from build123d import *
from OCP.BRepFilletAPI import BRepFilletAPI_MakeChamfer

# Parameters (mm, degrees)
SKETCH_1_R          = 2.85
EXTRUDE_1_DEPTH     = 1.4
FILLET_1_R          = 1.4
SKETCH_3_R          = 1.5
EXTRUDE_3_DEPTH     = 8
CUT_EXTRUDE_1_DEPTH = 1
CHAMFER_2_SIZE      = 0.3
CHAMFER_3_SIZE      = 0.576368876
CHAMFER_3_SIZE2     = 0.998300177
FILLET_2_R          = 0.1


with BuildPart() as part:
    # 草图1 → 凸台-拉伸1 (new body)
    with BuildSketch(Plane.XY):
        Circle(SKETCH_1_R)
    extrude(amount=EXTRUDE_1_DEPTH)

    # 圆角1
    fillet_1_edges = [part.edges().sort_by_distance(p)[0] for p in [
        (-2.85, 0, 1.4),
    ]]
    fillet(fillet_1_edges, radius=FILLET_1_R - 0.0001)  # a hair under: the kernel refuses the full size

    # 草图3 → 凸台-拉伸3 (add)
    with BuildSketch(Plane(origin=(0, 0, 0), x_dir=(-1, 0, 0), z_dir=(0, 0, -1))):
        with Locations(Location((0, 0, 0), (0, 0, 180))):
            Circle(SKETCH_3_R)
    extrude(amount=EXTRUDE_3_DEPTH)

    # 草图4 → 切除-拉伸1 (cut)
    with BuildSketch(Plane.XY.offset(1.4)):
        Polygon((1, 0.577350269), (0, 1.154700538), (-1, 0.577350269), (-1, -0.577350269), (0, -1.154700538), (1, -0.577350269), align=None)
    extrude(amount=-CUT_EXTRUDE_1_DEPTH, mode=Mode.SUBTRACT)

    # 倒角2
    chamfer_2_edges = [part.edges().sort_by_distance(p)[0] for p in [
        (-1.5, 0, -8),
    ]]
    chamfer(chamfer_2_edges, length=CHAMFER_2_SIZE)

    # 倒角3: one chamfer whose edges measure the first distance from different faces: ONE call of the kernel's chamfer builder (chamfer() names one face for all edges)
    chamfer_3_edges_1 = [part.edges().sort_by_distance(p)[0] for p in [
        (1, 0, 0.4),
    ]]
    chamfer_3_side_1 = [part.faces().sort_by_distance(p)[0] for p in [
        (1, 0, 0.9),
    ]]
    chamfer_3_edges_2 = [part.edges().sort_by_distance(p)[0] for p in [
        (0.5, -0.866025404, 0.4),
    ]]
    chamfer_3_side_2 = [part.faces().sort_by_distance(p)[0] for p in [
        (0.5, -0.866025404, 0.9),
    ]]
    chamfer_3_edges_3 = [part.edges().sort_by_distance(p)[0] for p in [
        (-0.5, -0.866025404, 0.4),
    ]]
    chamfer_3_side_3 = [part.faces().sort_by_distance(p)[0] for p in [
        (-0.5, -0.866025404, 0.9),
    ]]
    chamfer_3_edges_4 = [part.edges().sort_by_distance(p)[0] for p in [
        (-1, 0, 0.4),
    ]]
    chamfer_3_side_4 = [part.faces().sort_by_distance(p)[0] for p in [
        (-1, 0, 0.9),
    ]]
    chamfer_3_edges_5 = [part.edges().sort_by_distance(p)[0] for p in [
        (-0.5, 0.866025404, 0.4),
    ]]
    chamfer_3_side_5 = [part.faces().sort_by_distance(p)[0] for p in [
        (-0.5, 0.866025404, 0.9),
    ]]
    chamfer_3_edges_6 = [part.edges().sort_by_distance(p)[0] for p in [
        (0.5, 0.866025404, 0.4),
    ]]
    chamfer_3_side_6 = [part.faces().sort_by_distance(p)[0] for p in [
        (0.5, 0.866025404, 0.9),
    ]]
    chamfer_3 = BRepFilletAPI_MakeChamfer(part.part.solid().wrapped)
    for e in chamfer_3_edges_1:
        chamfer_3.Add(CHAMFER_3_SIZE, CHAMFER_3_SIZE2, e.wrapped, chamfer_3_side_1[0].wrapped)  # the first distance lies on this face
    for e in chamfer_3_edges_2:
        chamfer_3.Add(CHAMFER_3_SIZE, CHAMFER_3_SIZE2, e.wrapped, chamfer_3_side_2[0].wrapped)  # the first distance lies on this face
    for e in chamfer_3_edges_3:
        chamfer_3.Add(CHAMFER_3_SIZE, CHAMFER_3_SIZE2, e.wrapped, chamfer_3_side_3[0].wrapped)  # the first distance lies on this face
    for e in chamfer_3_edges_4:
        chamfer_3.Add(CHAMFER_3_SIZE, CHAMFER_3_SIZE2, e.wrapped, chamfer_3_side_4[0].wrapped)  # the first distance lies on this face
    for e in chamfer_3_edges_5:
        chamfer_3.Add(CHAMFER_3_SIZE, CHAMFER_3_SIZE2, e.wrapped, chamfer_3_side_5[0].wrapped)  # the first distance lies on this face
    for e in chamfer_3_edges_6:
        chamfer_3.Add(CHAMFER_3_SIZE, CHAMFER_3_SIZE2, e.wrapped, chamfer_3_side_6[0].wrapped)  # the first distance lies on this face
    add(Compound.cast(chamfer_3.Shape()), mode=Mode.REPLACE)

    # 圆角2
    fillet_2_edges = [part.edges().sort_by_distance(p)[0] for p in [
        (-1.5, 0, 0),
    ]]
    fillet(fillet_2_edges, radius=FILLET_2_R)


solid = part.part
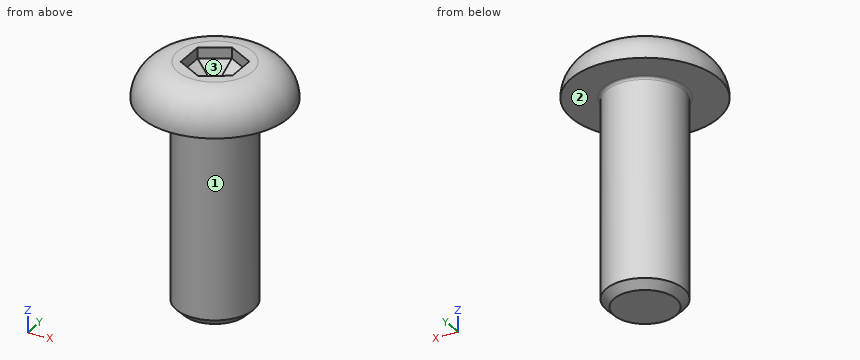
Geometry: final body of the model. Coordinates: model frame, mm. Face numbers are marked on the shaded views. Give positions to 0.01 mm unless a question says otherwise; leave off trailing zeros. Write each loop counter-clockwise with the first axis right and the second up, starting at its lowest first coordinate (ties: lowest second). Pieces come first, ordered by that corner, then holes. Notation, with made-up numbers: (-20.75, -8.5) -> (-3.75, -8.5) arc R23 cw to (-3.75, 23.5) -> close; hole circle Ø1 at (-35.75, 3). An arc over 180 degrees is marked (long way). Answer in a Markdown table with one row per item.
(1) Ray query, line 1 along Y through (x, z) = (0, -2.25); line 2 along X through (y, z) = (1.35, -2.5); line 3 along Z through (x, y) = (-0.35, -0.9). Return the intervals inside material, ascending. Write a range as [from, to].
Answers below:
| item | result |
|---|---|
| line 1 | [-1.5, 1.5] |
| line 2 | [-0.65, 0.65] |
| line 3 | [-8, 0.95] |
(2) Section query A-A on z = -5.25. Return loops of the section in (x, y).
Answers below:
| item | result |
|---|---|
| outline | circle Ø3 at (0, 0) |
(3) Draft query along X for the marked faces 1, 2 and 3. Return one class per face: +X half, -X half, draft (parallel to the pull), parting line (faces both ways), or undercut.
Answers below:
| item | result |
|---|---|
| face 1 | parting line |
| face 2 | draft |
| face 3 | undercut |
(4) Pin query (flat end, axial travel): pin 1 (2 mm diameter, centred on y = 1, z = -2, fed in from +X); pin 2 (2 mm diameter, centred on x = 2, z = -5, fed in from -Y). Return the tip coordinate at first contact, or that it passes through.
Answers below:
| item | result |
|---|---|
| pin 1 | x = 1.5 |
| pin 2 | y = -1.12 |
